Solid Edge part; units mm, degrees
sketch "Sketch1" plane through (0, 0, 0) normal (0, -1, 0) x (1, 0, 0)
  arc A0 (0, 2.032) -> (2.7813, 0.6773) centre (0, -1.5005) cw
  line L0 (2.7813, 0.6773) -> (2.7813, 0)
  line L1 (2.7813, 0) -> (1.5875, 0)
  line L2 (1.5875, 0) -> (1.5875, -5.9834)
  line L3 (1.5875, -5.9834) -> (0.9525, -6.35)
  line L4 (0.9525, -6.35) -> (0, -6.35)
  dimension "D1" = 2.7813
  dimension "D2" = 2.7813
  dimension "D3" = 2.7813
revolve "RevolvedProtrusion1" add sketch "Sketch1" angle 360 about axis through (0, 0, 0) along (0, 0, 1)
sketch "Sketch2" plane through (0, 0, 0.6773) normal (0, 0, 1) x (1, 0, 0)
  line L0 (0.4041, -0.4041) -> (1.5352, -0.4041)
  line L1 (1.5352, -0.4041) -> (1.5352, 0.4041)
  line L2 (1.5352, 0.4041) -> (0.4041, 0.4041)
  line L3 (0.4041, 0.4041) -> (0.4041, 1.5352)
  line L4 (0.4041, 1.5352) -> (-0.4041, 1.5352)
  line L5 (-0.4041, 1.5352) -> (-0.4041, 0.4041)
  line L6 (-0.4041, 0.4041) -> (-1.5352, 0.4041)
  line L7 (-1.5352, 0.4041) -> (-1.5352, -0.4041)
  line L8 (-1.5352, -0.4041) -> (-0.4041, -0.4041)
  line L9 (-0.4041, -0.4041) -> (-0.4041, -1.5352)
  line L10 (-0.4041, -1.5352) -> (0.4041, -1.5352)
  line L11 (0.4041, -1.5352) -> (0.4041, -0.4041)
extrude "Cutout1" cut sketch "Sketch2" along normal through all
cosmetic_thread "Thread1"
properties material "Acier galvanisé"
Part model, mm, in its own coordinate system. A direction names the side the tool comes from. Coordinates: 2 decimals unless noted, no trailing zeros. Loops run counter-clockwise (first coordinate to the right, second up) from the corner with the lowest first, then second, coordinate; pieces in that order, holes last. Notation, with made-up numbers: (-38, 10.25) -> (6, 10.25) arc R14 cw to (6, 25.25) -> close; hole circle Ø9 at (27.25, 35.5). An arc over 180 degrees is marked (long way). Use a Markdown table: item, result. Add a question column.
Item 1: Which spindle directions (+Z, -Z, +X, -X, +Y, -Y) get a long thin tool onto all of the face, cutting with end or side? Do faces 4 (the flat face through (0, 1.535, 1)), 5 (the cylindrical face through (2.569, 1.065, 0.334)). Say none if no direction does.
Item 2: Band-saw the part on C-C on z = -1. Write the cut outline in (x, y) (1 decimal), plus the area to 3 significant figures.
Item 3: Pull direction Y, two halves, no side cores. Call faces 1 (the flat face through (2, 0, 0)), 2 (the cylindrical face through (-0.34, 1.55, -3.03)), 3 (the flat face through (-0.404, -1, 1)): +Y half, -Y half, draft (parallel to the pull), parting line (faces both ways), or undercut.
Item 4: Probe probe 1 along Z at (x, y) = (0.45, -0.2); probe 2 along Z at (x, y) = (-0.1, -2.1); probe 3 along X at (y, z) = (-0.35, -2). List the from-to ranges inside material, lowest first.
Item 5: Band-saw the part on D-D on x = 1.95. Write the cut outline in (y, z), plus the area to 3 significant figures.
Item 6: Band-saw the part on A-A on y = 0. Write the cut outline in (x, z).
Item 7: Flat gauge pins, fed straight in: P1, Ø0.9, axis at x = -1, z = 1.5, coming from the -Y side; P2, Ø1, axis at y = 1.5, z = -3.5, coming from the +X side; P3, Ø1.2, axis at y = -1, z = 1.5, coming from the +X side. Where does each tip first touch, or does it go through?
Geometry says:
| question | item | result |
|---|---|---|
| 1 | face 4 | +Z |
| 1 | face 5 | +Z, -Z |
| 2 | outline | circle Ø3.2 at (0, 0) |
| 2 | area | 7.92 mm² |
| 3 | face 1 | draft |
| 3 | face 2 | parting line |
| 3 | face 3 | undercut |
| 4 | probe 1 | -6.35 to 0.68 |
| 4 | probe 2 | 0 to 1.34 |
| 4 | probe 3 | -1.55 to 1.55 |
| 5 | outline | (-1.98, 0) -> (1.98, 0) -> (1.98, 0.68) arc R2.95 ccw to (-1.98, 0.68) -> close |
| 5 | area | 4.78 mm² |
| 6 | outline | (-2.78, 0) -> (-1.59, 0) -> (-1.59, -5.98) -> (-0.95, -6.35) -> (0.95, -6.35) -> (1.59, -5.98) -> (1.59, 0) -> (2.78, 0) -> (2.78, 0.68) arc R3.53 ccw to (1.54, 1.68) -> (1.54, 0.68) -> (-1.54, 0.68) -> (-1.54, 1.68) arc R3.53 ccw to (-2.78, 0.68) -> close |
| 7 | P1 | y = -2.26 |
| 7 | P2 | x = 1.23 |
| 7 | P3 | x = 2.43 |
